Could you check a few things on this model? Use its own coordinates, in mm. Face numbers are marked on the shaded views. A direction names the side the tool comes from. Give positions to 0.01 mm unless a question says otherwise; leave off trailing zeros. Order: outer loops, then holes, each group sorted by start corner. A loop starts at its lowest first (then second) coordinate and runs counter-clockwise, first axis right, second up. Notation, with made-up numbers: (87, 3.5) -> (137, 3.5) arc R20 cw to (137, 29.5) -> close; hole circle Ø9 at (19.5, 51). An arc over 180 degrees is marked (long way). One line per item, written item: value.
Autodesk Inventor part; units mm, degrees
ref_plane "Work Plane1" through (0, 0, 25) normal (0, 0, 1) x (1, 0, 0)
ref_plane "Work Plane2" through (0, 0, 12.5) normal (0, 0, 1) x (1, 0, 0)
ref_plane "YZ Plane" through (0, 0, 0) normal (1, 0, 0) x (0, 1, 0)
sketch "Sketch1" plane through (0, 0, 0) normal (0, 0, 1) x (1, 0, 0)
  line L0 (0, 0) -> (0, 7.5)
  line L1 (0, 7.5) -> (20, 7.5)
  line L2 (20, 7.5) -> (20, 5)
  line L3 (20, 5) -> (30, 5)
  line L4 (30, 5) -> (30, 0)
  line L5 (30, 0) -> (0, 0)
  dimension "d0" = 30
  dimension "d1" = 10
  dimension "d2" = 15
  dimension "d3" = 10
revolve "Revolution1" add sketch "Sketch1" angle 360 about axis through (30, 0, 0) along (-1, 0, 0)
ref_plane "Work Plane1" through (0, 0, 25) normal (0, 0, 1) x (1, 0, 0)
sketch "Sketch2" plane through (0, 0, 25) normal (0, 0, 1) x (1, 0, 0)
  circle A0 centre (10, 0) radius 5
  point P0 (0, 0)
  dimension "d6" = 10
  dimension "d7" = 10
extrude "Extrusion1" add sketch "Sketch2" against normal up to surface
ref_plane "Work Plane2" through (0, 0, 12.5) normal (0, 0, 1) x (1, 0, 0)
sketch "Sketch3" plane through (0, 0, 12.5) normal (0, 0, 1) x (1, 0, 0)
  spline S0 degree 5 poles (15, 0) (15, 0.4219) (14.9555, 0.8387) (14.8687, 1.2398) (14.7463, 1.6158) (14.3477, 2.5523) (14.0183, 3.0596) (13.6471, 3.4841) (13.2419, 3.8427) (12.55, 4.312) (12.2828, 4.4645) (12.0061, 4.5954) (11.7208, 4.7045) (11.1518, 4.8741) (10.869, 4.9367) (10.5813, 4.9788) (10.2907, 5) (9.7153, 5) (9.4311, 4.9798) (9.1493, 4.9393) (8.8717, 4.8792) (8.3043, 4.7138) (8.0156, 4.6048) (7.7353, 4.4738) (7.4645, 4.3208) (6.884, 3.9294) (6.5801, 3.6794) (6.2931, 3.3932) (6.0271, 3.0673) (5.633, 2.4524) (5.4882, 2.1871) (5.3591, 1.9015) (5.2496, 1.5959) (5.0609, 0.8779) (4.9924, 0.4546) (4.9713, 0.0174) (4.9997, -0.4169) (5.1096, -1.0686) (5.1632, -1.2988) (5.2289, -1.5209) (5.305, -1.7336) (5.509, -2.2194) (5.6454, -2.4831) (5.7955, -2.7277) (5.957, -2.9541) (6.3184, -3.3966) (6.521, -3.6087) (6.7335, -3.8013) (6.9549, -3.9755) (7.4457, -4.3099) (7.7178, -4.4651) (7.9996, -4.5981) (8.29, -4.7088) (8.8615, -4.877) (9.1415, -4.9382) (9.4259, -4.9794) (9.7127, -5) (10.2898, -5) (10.5796, -4.979) (10.8666, -4.9371) (11.1485, -4.8748) (11.7152, -4.7064) (11.9989, -4.5984) (12.2741, -4.4688) (12.5399, -4.3179) (13.116, -3.9294) (13.4199, -3.6794) (13.7069, -3.3932) (13.973, -3.0673) (14.367, -2.4524) (14.5118, -2.1871) (14.6409, -1.9015) (14.7504, -1.5959) (14.8987, -1.0314) (14.9486, -0.7812) (14.9828, -0.5236) (15, -0.2621) (15, 0) knots 0 0 0 0 0 0 0.052953 0.052953 0.052953 0.052953 0.144858 0.144858 0.144858 0.144858 0.19905 0.19905 0.19905 0.19905 0.250146 0.250146 0.250146 0.250146 0.300195 0.300195 0.300195 0.300195 0.355044 0.355044 0.355044 0.355044 0.42274 0.42274 0.42274 0.42274 0.467615 0.467615 0.467615 0.467615 0.521968 0.521968 0.521968 0.521968 0.553072 0.553072 0.553072 0.553072 0.596617 0.596617 0.596617 0.596617 0.645101 0.645101 0.645101 0.645101 0.700146 0.700146 0.700146 0.700146 0.75049 0.75049 0.75049 0.75049 0.801269 0.801269 0.801269 0.801269 0.854949 0.854949 0.854949 0.854949 0.922334 0.922334 0.922334 0.922334 0.967006 0.967006 0.967006 0.967006 1 1 1 1 1 1
  line L0 (0, 7.5) -> (0, -7.5)
  line L1 (20, 7.5) -> (20, -7.5)
  line L2 (3.5, 0) -> (6.75, 5.6292)
  line L3 (6.75, 5.6292) -> (13.25, 5.6292)
  line L4 (13.25, 5.6292) -> (16.5, 0)
  line L5 (16.5, 0) -> (13.25, -5.6292)
  line L6 (13.25, -5.6292) -> (6.75, -5.6292)
  line L7 (6.75, -5.6292) -> (3.5, 0)
  point P0 (0, 0)
  point P1 (10, 0)
  dimension "d11" = 13
  dimension "d12" = 10
extrude "Extrusion2" add sketch "Sketch3" along normal mid plane 4
chamfer "Chamfer1" distance 1 angle 45 1 edges at (5.0001, 0.0275, 7.4999)
sketch "Sketch4" plane through (10, 0, 25) normal (0, 0, 1) x (1, 0, 0)
  circle A0 centre (0, 0) radius 5
  point P0 (-10, 0)
hole "Hole1" at (10, 0, 25) direction (0, 0, -1) diameter 5 depth 25
sketch "Sketch5" plane through (0, 0, 0) normal (-1, 0, 0) x (0, 0, 1)
  circle A0 centre (0, 0) radius 7.5
hole "Hole2" at (0, 0, 0) direction (1, 0, 0) diameter 8 depth 16
sketch "Sketch6" plane through (30, 0, 0) normal (1, 0, 0) x (0, 0, -1)
  circle A0 centre (0, 0) radius 5
hole "Hole3" at (30, 0, 0) direction (-1, 0, 0) diameter 6 depth 14
thread "Thread2"
sketch "Sketch7" plane through (0, 0, 14.5) normal (0, 0, 1) x (1, 0, 0)
  circle A0 centre (10, 0) radius 2.5
  line L0 (6.75, -5.6292) -> (3.5, 0)
  line L1 (3.5, 0) -> (6.75, 5.6292)
  line L2 (6.75, 5.6292) -> (13.25, 5.6292)
  line L3 (13.25, 5.6292) -> (16.5, 0)
  line L4 (16.5, 0) -> (13.25, -5.6292)
  line L5 (13.25, -5.6292) -> (6.75, -5.6292)
  circle A1 centre (10, 0) radius 5
  circle A2 centre (10, 0) radius 5.5
  point P0 (0, 0)
  dimension "d43" = 11
extrude "Extrusion3" add sketch "Sketch7" along normal blind 1 contours A2
thread "Thread3"
thread "Thread4"
properties part number "123"
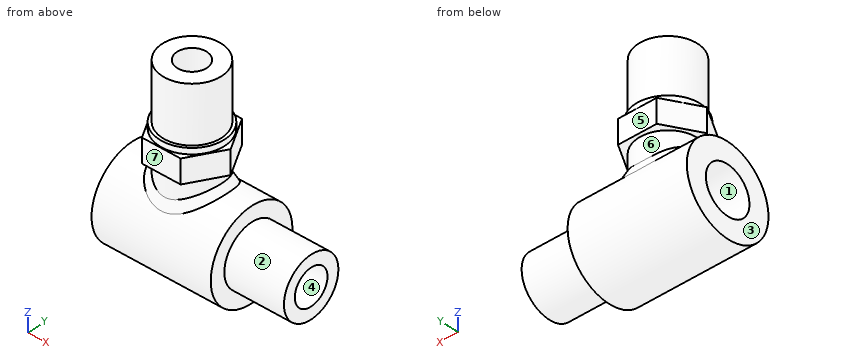
1) Suppose I cut it at B-B, the plane x = 3. Write out the boundary of the cut face in (y, z).
Answer below:
outline: circle Ø15 at (0, 0); hole circle Ø8 at (0, 0)
2) For the marked faces 5, 6 and 7, which set-ups out of +Z, -Z, +X, -X, +Y, -Y let a thin tool reach every point of the face, with its end or its side?
Answer below:
face 5: +Z, +X, -X, +Y
face 6: none
face 7: +Z, +X, -X, -Y
3) Suppose I cut it at D-D, the plane x = 19. Write out the boundary of the cut face in (y, z), then the cut area to 3 significant figures.
Answer below:
outline: circle Ø15 at (0, 0); hole circle Ø6 at (0, 0)
area: 148 mm2
4) Suppose I cut it at C-C, the plane y = -1.25. State how many separate pieces and enclosed holes the cut face has, then the cut area to 3 significant figures.
Answer below:
separate pieces: 3
enclosed holes: 0
area: 283 mm2
5) Suppose I cut it at A-A, the plane z = 0. Write out the boundary of the cut face in (x, y).
Answer below:
outline: (0, -7.5) -> (20, -7.5) -> (20, -5) -> (30, -5) -> (30, -3) -> (16, -3) -> (16, -4) -> (0, -4) -> close; (0, 4) -> (16, 4) -> (16, 3) -> (30, 3) -> (30, 5) -> (20, 5) -> (20, 7.5) -> (0, 7.5) -> close
6) For P1, Ø5, axis at y = 1.5, z = 14, coming from the +X side; P2, Ø2, axis at x = 9.5, z = 12.5, coming from the +Y side; P3, Ø1, axis at x = 24.5, y = 3.5, coming from the +Z side; P4, Ø3.5, axis at y = 0, z = 0, coming from the +X side, each with a flat end and sliding along its axis, tell me the tip position at first contact or that it passes through.
Answer below:
P1: stops at x = 16.5
P2: stops at y = 5.63
P3: stops at z = 4
P4: passes through
7) We'd pull the mould along Z, two halves only. Please class the marked faces 1, 2, 3 and 4: +Z half, -Z half, draft (parallel to the pull), parting line (faces both ways), or undercut.
Answer below:
face 1: undercut
face 2: parting line
face 3: draft
face 4: undercut
8) If I drill on line 1 along Y through (x, z) = (10, 18); line 2 along Z through (x, y) = (4.5, -1); line 3 along Y through (x, z) = (10.75, 0), over which ranges is the centre line in solid material (lowest first)?
Answer below:
line 1: y = -5 to -2.5, 2.5 to 5
line 2: z = -7.43 to -3.87, 3.87 to 7.85, 10.5 to 14.5
line 3: y = -7.5 to -4, 4 to 7.5
